```python
from build123d import *

# Parameters (mm, degrees)
BOSS_EXTRUDE1_DEPTH = 3.18
SKETCH2_R           = 1.6
CUT_EXTRUDE1_DEPTH  = 3.18
SKETCH3_R           = 1.6
CUT_EXTRUDE2_DEPTH  = 10


with BuildPart() as part:
    # Sketch1 → Boss-Extrude1 (new body)
    with BuildSketch(Plane(origin=(0, 0, 0), x_dir=(1, 0, 0), z_dir=(0, 1, 0))):
        Polygon((0, 0), (-55, 47.5), (-55, -47.5), align=None)
        Polygon((55, -47.5), (0, 0), (-55, -47.5), align=None)
        Polygon((55, 47.5), (0, 0), (55, -47.5), align=None)
        Polygon((55, 47.5), (-55, 47.5), (0, 0), align=None)
    extrude(amount=BOSS_EXTRUDE1_DEPTH)

    # Sketch2 → Cut-Extrude1 (cut)
    with BuildSketch(Plane(origin=(0, 3.18, 0), x_dir=(1, 0, 0), z_dir=(0, 1, 0))):
        with Locations((-20.4, 25.25)):
            Circle(SKETCH2_R)
        with Locations((-22, -23.05)):
            Circle(SKETCH2_R)
        with Locations((30.4, 9.95)):
            Circle(SKETCH2_R)
        with Locations((30.4, -17.95)):
            Circle(SKETCH2_R)
    extrude(amount=-CUT_EXTRUDE1_DEPTH, mode=Mode.SUBTRACT)

    # Sketch3 → Cut-Extrude2 (cut)
    with BuildSketch(Plane(origin=(0, 3.18, 0), x_dir=(1, 0, 0), z_dir=(0, 1, 0))):
        with Locations((45, 37.5)):
            Circle(SKETCH3_R)
        with Locations((45, -37.5)):
            Circle(SKETCH3_R)
        with Locations((-45, 37.5)):
            Circle(SKETCH3_R)
        with Locations((-45, -37.5)):
            Circle(SKETCH3_R)
    extrude(amount=-CUT_EXTRUDE2_DEPTH, mode=Mode.SUBTRACT)


solid = part.part
```
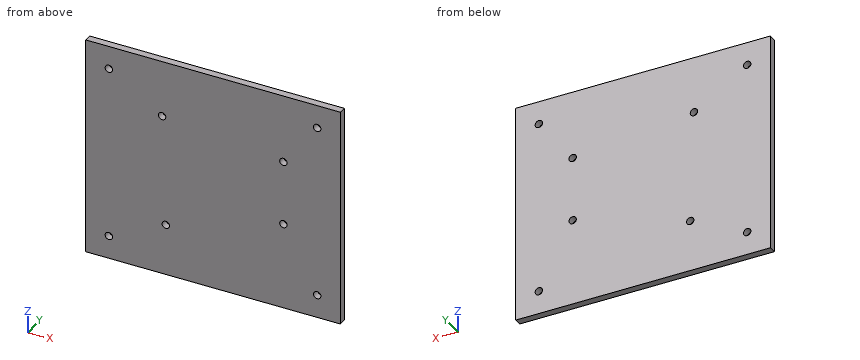
Input: part model. Units: mm. Frame: model coordinates. Coordinates: 2 decimals unless noted, no trailing zeros. Order: outer loops, then holes, each group sorted by start corner. A loop starts at its lowest first (then second) coordinate and runs counter-clockwise, first axis right, second up. Notation, with made-up numbers: (46, 21) - (60, 21) arc R20 ccw to (60, 41) - close; hole circle Ø10 at (-33.75, -23). An arc over 180 degrees is marked (long way). Return JSON: item names as keys, results as strings.
Q1. Ray query, probe 1 along Z at (x, y) = (-45, 2.05); probe 2 along X at (y, z) = (1.25, -9.95); probe 3 along X at (y, z) = (1.35, -25.25). Return the intervals inside material, ascending.
The answers:
{"probe 1": "z = -47.5 to -39.1, -35.9 to 35.9, 39.1 to 47.5", "probe 2": "x = -55 to 28.8, 32 to 55", "probe 3": "x = -55 to -22, -18.8 to 55"}
Q2. Cut plane C-C (z = 17.95). Return loops of the section in (x, y).
The answers:
{"outline": "(-55, 0) - (28.8, 0) - (28.8, 3.18) - (-55, 3.18) - close; (32, 0) - (55, 0) - (55, 3.18) - (32, 3.18) - close"}
Q3. Cut plane A-A (x = 45). Return loops of the section in (y, z).
The answers:
{"outline": "(0, -47.5) - (3.18, -47.5) - (3.18, -39.1) - (0, -39.1) - close; (0, -35.9) - (3.18, -35.9) - (3.18, 35.9) - (0, 35.9) - close; (0, 39.1) - (3.18, 39.1) - (3.18, 47.5) - (0, 47.5) - close"}
Q4. Cut plane B-B (z = 37.5). Return loops of the section in (x, y).
The answers:
{"outline": "(-55, 0) - (-46.6, 0) - (-46.6, 3.18) - (-55, 3.18) - close; (-43.4, 0) - (43.4, 0) - (43.4, 3.18) - (-43.4, 3.18) - close; (46.6, 0) - (55, 0) - (55, 3.18) - (46.6, 3.18) - close"}
